Geometry check sheet. Reference: the model listing, model coordinates, mm. A direction names the side the tool comes from. Coordinates: 2 decimals unless noted, no trailing zeros. Write each loop counter-clockwise with the first axis right and the second up, starting at its lowest first coordinate (ties: lowest second). Pieces come first, ordered by that corner, then holes. Notation, with made-up numbers: M 40.25,-33.5 L 55.25,-33.5 A17 ccw 55.25,-6.5 Z; hole C 54.25,83 d10. An arc over 180 degrees is marked long. Put each result on its own line as item: value. Start each with the question number.
1) Scan lines: line 1 along Y through (x, z) = (21, 2.3); line 2 along Y through (x, z) = (-21, 1.05); line 3 along Y through (x, z) = (14.5, 2.7). Record each from-to range of solid material in increasing order.
2) Cross-section at A-A on x = 21. Record the cut outline in (y, z), plus the area to 3 significant figures.
3) Mould release check, pull along Y, two halves, no side actions. Record for faces 1 (the flat face through (0, 19.5, 1)), 2 (the cylindrical face through (19.712, 17.406, 1.479)), 3 (the flat face through (23.5, 11, 1)), 4 (the flat face through (0, -19.5, 1)): released by +Y, released by -Y, zero draft, split by the parting line, or undercut.
4) Gauge pin test, flat end, axial feed: pin 1 (1.6 mm diameter, centred on x = -21, y = -17, fed in from +Z). Record the tip position at first contact, or that the pin passes through.
5) Cross-section at C-C on z = 1.3. Record the cut outline in (x, y), plus the area to 3 significant figures.
6) Cross-section at D-D on x = 13. Record the cut outline in (y, z).
7) Cross-section at B-B on y = -17. Record the cut outline in (x, z).
8) Set-up check for faces 5 (the flat face through (15, -3, 2)), 6 (the flat face through (-23.5, 0, 1)): record each of +Z, -Z, +X, -X, +Y, -Y from which the full face is reachable in a straight line by a thin tool's end or side.
from build123d import *

# Parameters (mm, degrees)
SKETCH_1_W           = 47
SKETCH_1_H           = 39
EXTRUDE_1_DEPTH      = 3
HOLE_WIZARD_M2_5_1_D = 2.7
CUT_EXTRUDE_1_REACH  = 32.684


with BuildPart() as part:
    # 草图1 → 凸台-拉伸1 (new body)
    with BuildSketch(Plane.XY):
        Rectangle(SKETCH_1_W, SKETCH_1_H)
    extrude(amount=EXTRUDE_1_DEPTH)

    # M2.5 间隙孔1 (through all)
    with Locations(Plane.XY.offset(3)):
        with Locations((-21, -17), (21, 17), (21, -17), (-21, 17)):
            Hole(HOLE_WIZARD_M2_5_1_D / 2)

    # 草图5 → 切除-拉伸1 (cut, up to next)
    with BuildSketch(Plane.XY.offset(3), mode=Mode.PRIVATE) as cut_extrude_1_sk1:
        with BuildLine():
            Line((6.5, 3), (23.5, 3))
            ThreePointArc((23.5, 3), (26.5, 0), (23.5, -3))
            Line((23.5, -3), (6.5, -3))
            ThreePointArc((6.5, -3), (3.5, 0), (6.5, 3))
        make_face()
    cut_extrude_1_tool1 = extrude(cut_extrude_1_sk1.sketch, amount=-CUT_EXTRUDE_1_REACH, mode=Mode.PRIVATE) & part.part
    add(cut_extrude_1_tool1.solids().sort_by_distance((15, 0, 3))[0], mode=Mode.SUBTRACT)


solid = part.part
Answer key:
1. line 1: y = -19.5 to -18.35, -15.65 to -3, 3 to 15.65, 18.35 to 19.5
1. line 2: y = -19.5 to -18.35, -15.65 to 15.65, 18.35 to 19.5
1. line 3: y = -19.5 to -3, 3 to 19.5
2. outline: M -19.5,0 L -18.35,0 L -18.35,3 L -19.5,3 Z; M -15.65,0 L -3,0 L -3,3 L -15.65,3 Z; M 3,0 L 15.65,0 L 15.65,3 L 3,3 Z; M 18.35,0 L 19.5,0 L 19.5,3 L 18.35,3 Z
2. area: 82.8 mm²
3. face 1: released by +Y
3. face 2: undercut
3. face 3: zero draft
3. face 4: released by -Y
4. pin 1: passes through
5. outline: M -23.5,-19.5 L 23.5,-19.5 L 23.5,-3 L 6.5,-3 A3 cw 6.5,3 L 23.5,3 L 23.5,19.5 L -23.5,19.5 Z; hole C -21,-17 d2.7; hole C -21,17 d2.7; hole C 21,-17 d2.7; hole C 21,17 d2.7
5. area: 1,690 mm²
6. outline: M -19.5,0 L -3,0 L -3,3 L -19.5,3 Z; M 3,0 L 19.5,0 L 19.5,3 L 3,3 Z
7. outline: M -23.5,0 L -22.35,0 L -22.35,3 L -23.5,3 Z; M -19.65,0 L 19.65,0 L 19.65,3 L -19.65,3 Z; M 22.35,0 L 23.5,0 L 23.5,3 L 22.35,3 Z
8. face 5: +Z, -Z, +X
8. face 6: +Z, -Z, -X, +Y, -Y
